Check sheet for the modelled part. Datum: model origin and axes. Units: mm. A direction names the side the tool comes from. Give positions to 0.01 mm unless a question says otherwise; leave off trailing zeros. Loops run counter-clockwise (first coordinate to the right, second up) from the corner with the lowest first, then second, coordinate; pieces in that order, holes last. Notation, with made-up numbers: (-16.75, 57.25) -> (-1.75, 57.25) arc R19 ccw to (-1.75, 90.25) -> close; hole circle Ø9 at (-40, 1). An arc over 180 degrees is marked (long way). Write each question's results on one line, items separated by ' | '. Start each with the question number.
Item 1: Cross-section at B-B on z = -51. Enter the section's corners in (x, y).
Item 2: Scan lines: line 1 along Z through (x, y) = (0, 2.6); line 2 along Z through (x, y) = (2, 1.25); line 3 along Y through (x, z) = (-6.5, -46). Record each from-to range of solid material in increasing order.
Item 3: Mould release check, pull along X, two halves, no side actions. Record for faces 1 (the face through (-5, 10, 2)), 2 (the face through (10, 5, 2)), 3 (the face through (1.4, 1.86, 57.81)): pulls with the +X half, pulls with the -X half, needs draft (parallel to the pull), parting line crosses it, or undercut.
Item 4: Access from +Z, -Z, +X, -X, +Y, -Y to the whole of each face (thin tool, end or side, straight path). Record for faces 4 (the face through (0, 3.6, 1)), 5 (the face through (0, 3, -112.5)).
Item 5: Gauge pin test, flat ends, axial feed: pin 1 Ø2.5 at (x, y) = (6.5, 3.5) entering from +Z; pin 2 Ø3.5 at (x, z) = (-1, -26.5) entering from +Y; pin 3 Ø1.4 at (x, z) = (0, 77.5) entering from +Y; pin 4 Ø1 at (y, z) = (8, 47) entering from +X. Record the tip position at first contact, or that the pin passes through.
Item 6: Cross-section at A-A on x = 0. Enter the section's corners in (y, z).
from build123d import *

# Parameters (mm, degrees)
SKETCH1_R            = 1.65
BOSS_EXTRUDE1_DEPTH  = 112.5
M5_CLEARANCE_HOLE1_D = 5.2


with BuildPart() as part:
    # Sketch1 → Boss-Extrude1 (new, symmetric)
    with BuildSketch(Plane.XY):
        with BuildLine():
            Line((-7, 10), (-3.35, 10))
            ThreePointArc((-3.35, 10), (-2.819669914, 9.780330086), (-2.6, 9.25))
            Line((-2.6, 9.25), (-2.6, 8.45))
            ThreePointArc((-2.6, 8.45), (-2.673223305, 8.273223305), (-2.85, 8.2))
            Line((-2.85, 8.2), (-5.389339828, 8.2))
            ThreePointArc((-5.389339828, 8.2), (-6.082249478, 7.737012574), (-5.919669914, 6.919669914))
            Line((-5.919669914, 6.919669914), (-2.819669914, 3.819669914))
            ThreePointArc((-2.819669914, 3.819669914), (-2.576352402, 3.657090351), (-2.289339828, 3.6))
            Line((-2.289339828, 3.6), (2.289339828, 3.6))
            ThreePointArc((2.289339828, 3.6), (2.576352402, 3.657090351), (2.819669914, 3.819669914))
            Line((2.819669914, 3.819669914), (5.919669914, 6.919669914))
            ThreePointArc((5.919669914, 6.919669914), (6.082249478, 7.737012574), (5.389339828, 8.2))
            Line((5.389339828, 8.2), (2.85, 8.2))
            ThreePointArc((2.85, 8.2), (2.673223305, 8.273223305), (2.6, 8.45))
            Line((2.6, 8.45), (2.6, 9.25))
            ThreePointArc((2.6, 9.25), (2.819669914, 9.780330086), (3.35, 10))
            Line((3.35, 10), (7, 10))
            ThreePointArc((7, 10), (9.121320344, 9.121320344), (10, 7))
            Line((10, 7), (10, 3))
            ThreePointArc((10, 3), (9.121320344, 0.878679656), (7, 0))
            Line((7, 0), (-7, 0))
            ThreePointArc((-7, 0), (-9.121320344, 0.878679656), (-10, 3))
            Line((-10, 3), (-10, 7))
            ThreePointArc((-10, 7), (-9.121320344, 9.121320344), (-7, 10))
        make_face()
        with Locations((-6.5, 3.5)):
            Circle(SKETCH1_R, mode=Mode.SUBTRACT)
        with Locations((6.5, 3.5)):
            Circle(SKETCH1_R, mode=Mode.SUBTRACT)
    extrude(amount=BOSS_EXTRUDE1_DEPTH, both=True)

    # M5 Clearance Hole1 (through all)
    with Locations(Plane(origin=(0, 0, 0), x_dir=(-1, 0, 0), z_dir=(0, -1, 0))):
        with Locations((0, 60), (0, -60)):
            Hole(M5_CLEARANCE_HOLE1_D / 2)


solid = part.part
Answer sheet:
1) outline: (-10, 3) arc R3 ccw to (-7, 0) -> (7, 0) arc R3 ccw to (10, 3) -> (10, 7) arc R3 ccw to (7, 10) -> (3.35, 10) arc R0.75 ccw to (2.6, 9.25) -> (2.6, 8.45) arc R0.25 ccw to (2.85, 8.2) -> (5.39, 8.2) arc R0.75 cw to (5.92, 6.92) -> (2.82, 3.82) arc R0.75 cw to (2.29, 3.6) -> (-2.29, 3.6) arc R0.75 cw to (-2.82, 3.82) -> (-5.92, 6.92) arc R0.75 cw to (-5.39, 8.2) -> (-2.85, 8.2) arc R0.25 ccw to (-2.6, 8.45) -> (-2.6, 9.25) arc R0.75 ccw to (-3.35, 10) -> (-7, 10) arc R3 ccw to (-10, 7) -> close; hole circle Ø3.3 at (-6.5, 3.5); hole circle Ø3.3 at (6.5, 3.5)
2) line 1: z = -112.5 to -62.6, -57.4 to 57.4, 62.6 to 112.5 | line 2: z = -112.5 to -61.66, -58.34 to 58.34, 61.66 to 112.5 | line 3: y = 0 to 1.85, 5.15 to 10
3) face 1: needs draft | face 2: pulls with the +X half | face 3: undercut
4) face 4: +Z, -Z, +Y | face 5: -Z, +X, -X, +Y, -Y
5) pin 1: passes through | pin 2: stops at y = 9.7 | pin 3: stops at y = 3.6 | pin 4: stops at x = 9.96
6) outline: (0, -112.5) -> (3.6, -112.5) -> (3.6, -62.6) -> (0, -62.6) -> close; (0, -57.4) -> (3.6, -57.4) -> (3.6, 57.4) -> (0, 57.4) -> close; (0, 62.6) -> (3.6, 62.6) -> (3.6, 112.5) -> (0, 112.5) -> close
